Geometry check sheet. Reference: drawing and pictorial views, mm from the part's lowest x, y, z. Round coordinates to 2 decimals unless told otherwise and drop trailing zeros. Write each loop counter-clockwise with the first axis right and the second up, starting at its lowest first coordinate (ties: lowest second). Pieces come first, ordered by that corner, then holes. Notation, with made-up numbers: (-26, 16) -> (10, 16) arc R28 cw to (10, 43) -> close; hole circle Ø10 at (-8, 14). An arc over 180 degrees is marked (long way). Answer as a JSON object with one key per item and string values. Group by question number.
(1) Gauge pin test, flat ends, axial feed: pin 1 Ø2 at (x, z) = (1.5, 86.5) entering from -Y; pin 2 Ø2 at (x, y) = (2.5, 9.5) entering from -Z (1 decimal); pin 3 Ø2 at (x, y) = (2, 9) entering from -Z (1 decimal). Record the tip position at first contact, or that the pin passes through.
(2) Scan lines: L1, parallel to Z at x = 3.65, y = 42.5 (1 decimal); L2, parallel to Z at x = 0.2, y = 40 (1 decimal); L3, parallel to Y at x = 0.3, z = 44. Record each from-to range of solid material in increasing order. Write a range as from..to.
(3) Sectioned sample at B-B on z = 45.5. Record the cut outline in (x, y).
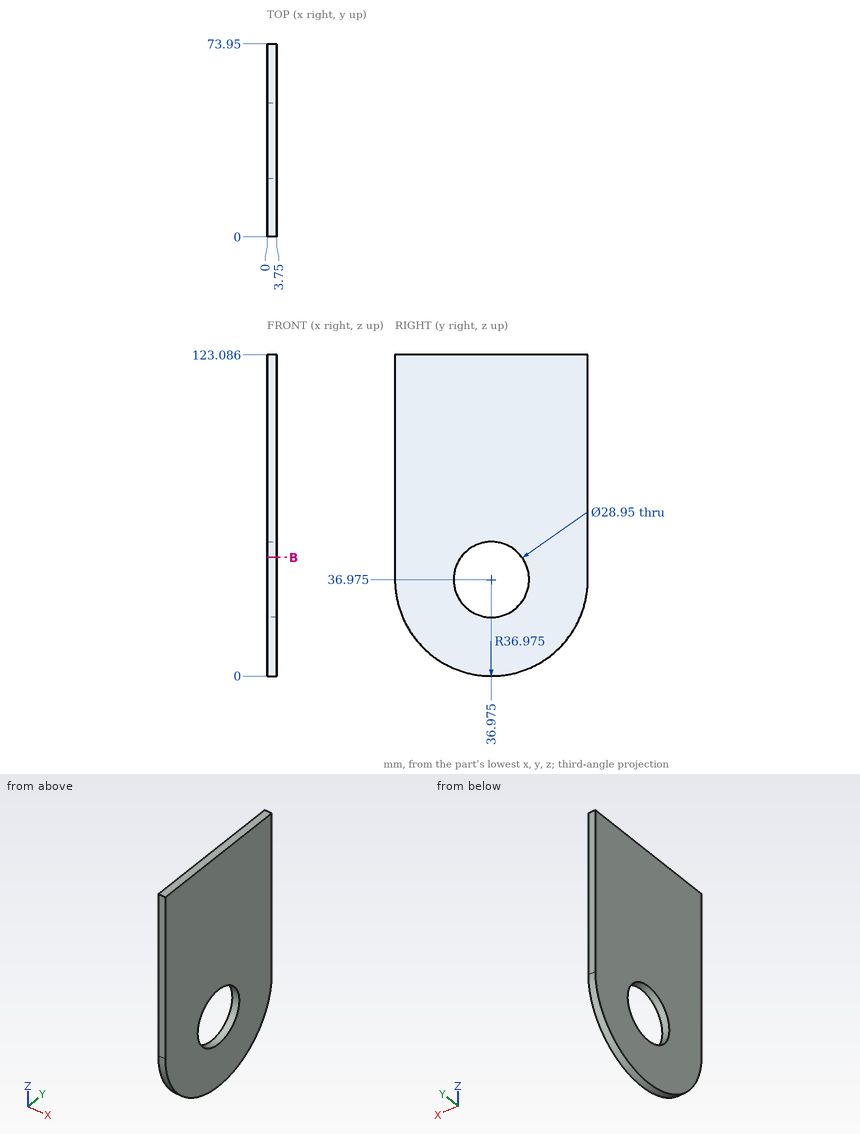
Computed values:
{
 "1": {"pin 1": "y = 0", "pin 2": "z = 11.2", "pin 3": "z = 11.7"},
 "2": {"L1": "0.4..23.6, 50.4..123.1", "L2": "0.1..22.8, 51.1..123.1", "L3": "0..24.32, 49.63..73.95"},
 "3": {"outline": "(0, 0) -> (3.75, 0) -> (3.75, 25.28) -> (0, 25.28) -> close; (0, 48.67) -> (3.75, 48.67) -> (3.75, 73.95) -> (0, 73.95) -> close"}
}
